Read the model definition and answer for the solid it produces. Units are mm, in the model's axes. A direction names the side the tool comes from. Coordinates: 2 decimals unless noted, no trailing zeros. Order: outer loops, then holes, each group sorted by start corner. A loop starts at its lowest first (then second) coordinate and runs counter-clockwise, first axis right, second up. Notation, with made-up numbers: M 63,-35 L 96,-35 A10 cw 96,-18 Z; hole C 47.25,-21.75 d7. An arc over 180 degrees is marked long. Use a Markdown table: item, result. Add a question column.
1) Find section A-A on x = 0. Write down the section's boundary in (y, z).
2) For faces 5 (the face through (-37, 15, 38)), 6 (the face through (1, 29, 0)), determine the directions among +Z, -Z, +X, -X, +Y, -Y from which every point of the face is accessible in a straight line to the end or side of a thin tool.
3) Each of these flat-tipped pins is pushed along its axis until it touches: pin 1 Ø5.5 at (x, y) = (-32, 26.5) entering from +Z; pin 2 Ø8 at (x, z) = (26.5, 31) entering from -Y; pin 3 Ø12 at (x, z) = (18.5, 42.5) entering from -Y. Where does it stop, or does it pass through?
4) Find section B-B on y = 22. Write down the section's boundary in (x, z), plus the area to 3 significant figures.
5) Find section D-D on x = -27. Write down the section's boundary in (y, z), plus the area to 3 significant figures.
6) Find section C-C on z = 29. Write down the section's boundary in (x, y).
7) Find the intervals of material crossed by probe 1 along X at (y, z) = (34, 21); probe 2 along Y at (x, z) = (0, 10); probe 3 along Y at (x, z) = (27, 32), in increasing order. Write a range as [from, to].
8) The mould has two halves that part along Y. Classify faces 1 (the face through (28, 19, 26)), 2 (the face through (1, 57, 25)), 3 (the face through (7.63, 21.4, 8.11)), 4 (the face through (0.5, 10.8, 16)): released by +Y, released by -Y, zero draft, split by the parting line, or undercut.
from build123d import *

# Parameters (mm, degrees)
F1_DEPTH = 37
F2_W     = 36
F2_H     = 19
F3_DEPTH = 19
F4_W     = 57
F4_H     = 51
F5_DEPTH = 19
F6_W     = 57
F6_H     = 51
F7_DEPTH = 19
F8_R     = 8
F9_DEPTH = 51


with BuildPart() as f1:
    # F0 (on Right) → F1 (new body, symmetric)
    with BuildSketch(Plane.YZ):
        Polygon((0, 16), (0, 0), (57, 0), (57, 51), (38, 51), (38, 35), (19, 35), (19, 16), align=None)
    extrude(amount=F1_DEPTH, both=True)

    # F2 (on face) → F3 (cut)
    with BuildSketch(Plane.XY.offset(35)):
        with Locations((0, 28.5)):
            Rectangle(F2_W, F2_H)
    extrude(amount=-F3_DEPTH, mode=Mode.SUBTRACT)

    # F4 (on face) → F5 (join)
    with BuildSketch(Plane.YZ.offset(37)):
        with Locations((28.5, 25.5)):
            Rectangle(F4_W, F4_H)
    extrude(amount=F5_DEPTH)

    # F6 (on face) → F7 (join)
    with BuildSketch(Plane(origin=(-37, 0, 0), x_dir=(0, -1, 0), z_dir=(-1, 0, 0))):
        with Locations((-28.5, 25.5)):
            Rectangle(F6_W, F6_H)
    extrude(amount=F7_DEPTH)

    # F8 (on face) → F9 (cut)
    with BuildSketch(Plane.XY.offset(16)):
        with Locations((0, 19)):
            Circle(F8_R)
    extrude(amount=-F9_DEPTH, mode=Mode.SUBTRACT)


solid = f1.part
Check result:
| question | item | result |
|---|---|---|
| 1 | outline | M 0,0 L 11,0 L 11,16 L 0,16 Z; M 27,0 L 57,0 L 57,51 L 38,51 L 38,16 L 27,16 Z |
| 2 | face 5 | +Z, -Y |
| 2 | face 6 | -Z, +X, -X, +Y, -Y |
| 3 | pin 1 | stops at z = 35 |
| 3 | pin 2 | stops at y = 19 |
| 3 | pin 3 | stops at y = 38 |
| 4 | outline | M -56,0 L -7.42,0 L -7.42,16 L -18,16 L -18,35 L -37,35 L -37,51 L -56,51 Z; M 7.42,0 L 56,0 L 56,51 L 37,51 L 37,35 L 18,35 L 18,16 L 7.42,16 Z |
| 4 | area | 3,610 mm2 |
| 5 | outline | M 0,0 L 57,0 L 57,51 L 38,51 L 38,35 L 19,35 L 19,16 L 0,16 Z |
| 5 | area | 1,940 mm2 |
| 6 | outline | M -56,0 L -37,0 L -37,19 L -18,19 L -18,38 L 18,38 L 18,19 L 37,19 L 37,0 L 56,0 L 56,57 L -56,57 Z |
| 7 | probe 1 | x = [-56, -18], [18, 56] |
| 7 | probe 2 | y = [0, 11], [27, 57] |
| 7 | probe 3 | y = [19, 57] |
| 8 | face 1 | released by -Y |
| 8 | face 2 | released by +Y |
| 8 | face 3 | undercut |
| 8 | face 4 | zero draft |
